For this review, take the finished solid that the model builds, in its own axes (mm). A direction names the side the tool comes from. Round coordinates to 2 decimals unless told otherwise and drop trailing zeros. Loops run counter-clockwise (first coordinate to the right, second up) from the corner with the lowest first, then second, coordinate; pieces in that order, holes last.
1) Insertion check: pin 1 (0.9 mm diameter, centred on y = 19.5, z = 12.5, fed in from -X); pin 2 (10 mm diameter, centred on y = 12.5, z = 10, fed in from +X) (3 decimals); pin 3 (5 mm diameter, centred on x = 31, y = 14.5, fed in from +Z). Each pin has a flat end and moves straight along its axis. Give the tip position at first contact, or say it passes through.
2) Take a section at A-A (z = 26.5). State the section outline as (x, y) points.
3) Mouldability with a two-part tool opening along Z and no side actions: class faces 1 (the cylindrical face through (71, 20.5, 12.6)), 2 (the flat face through (53, 13, 0)), 3 (the flat face through (53, 0, 12)) as pulls with the +Z half, pulls with the -Z half, needs draft (parallel to the pull), parting line crosses it, or undercut.
4) Tool access review of faces 4 (the cylindrical face through (71, 4.5, 12.4)), 5 (the cylindrical face through (33, 20.5, 12.6)), 6 (the cylindrical face through (66.61, 9.44, 23.16)), 7 (the flat face through (74, 21, 35)): name each direction out of +Z, -Z, +X, -X, +Y, -Y from which nothing blocks a thin tool from reaching the whole face with its end or side.
5) Wall thickness on L1, parallel to X at y = 13, z = 23; L2, parallel to Y at x = 11, z = 12.5; L3, parallel to Y at x = -5, z = 12.5: over which ranges is each line inside the solid? List them lowest first.
6) Take a section at D-D (y = 12.5). Give the number of separate pieces and of enclosed holes in the cut face, then the cut area to 3 significant figures.
7) Take a section at B-B (x = 17). State the section outline as (y, z) points, then the cut area to 3 significant figures.
8) Take a section at C-C (x = 79.5). State the section outline as (y, z) points.
```python
from build123d import *

# Parameters (mm, degrees)
SZKIC1_W                    = 52
SZKIC1_H                    = 25
DODANIE_WYCI_GNI_CIE1_DEPTH = 25
SZKIC1_3_R                  = 10
DODANIE_WYCI_GNI_CIE2_DEPTH = 35
SZKIC2_R                    = 10
DODANIE_WYCI_GNI_CIE3_DEPTH = 15
SZKIC3_R                    = 8
WYTNIJ_WYCI_GNI_CIE1_DEPTH  = 50
SZKIC4_R                    = 8
WYTNIJ_WYCI_GNI_CIE2_DEPTH  = 31


with BuildPart() as part:
    # Szkic1 → Dodanie-wyci_gni_cie1 (new body)
    with BuildSketch(Plane.XY):
        with Locations((26, 12.5)):
            Rectangle(SZKIC1_W, SZKIC1_H)
    extrude(amount=DODANIE_WYCI_GNI_CIE1_DEPTH)

    # Szkic1_3 → Dodanie-wyci_gni_cie2 (add)
    with BuildSketch(Plane.XY):
        with Locations((30, 12.5)):
            Circle(SZKIC1_3_R)
    extrude(amount=DODANIE_WYCI_GNI_CIE2_DEPTH)

    # Szkic2 → Dodanie-wyci_gni_cie3 (add)
    with BuildSketch(Plane(origin=(0, 0, 0), x_dir=(0, 0, -1), z_dir=(1, 0, 0))):
        with Locations((-12.5, 12.5)):
            Circle(SZKIC2_R)
    extrude(amount=-DODANIE_WYCI_GNI_CIE3_DEPTH)

    # Szkic3 → Wytnij-wyci_gni_cie1 (cut)
    with BuildSketch(Plane.ZY.offset(15)):
        with Locations((12.5, 12.5)):
            Circle(SZKIC3_R)
    extrude(amount=-WYTNIJ_WYCI_GNI_CIE1_DEPTH, mode=Mode.SUBTRACT)

    # Szkic4 → Wytnij-wyci_gni_cie2 (cut)
    with BuildSketch(Plane.XY.offset(35)):
        with Locations((30, 12.5)):
            Circle(SZKIC4_R)
    extrude(amount=-WYTNIJ_WYCI_GNI_CIE2_DEPTH, mode=Mode.SUBTRACT)

    # Lustro1: part across plane


with BuildPart() as part_1:
    add(part.part)
    add(part.part.mirror(Plane(origin=(52, 0, 25), x_dir=(0, 0, 1), z_dir=(1, 0, 0))))


solid = part_1.part
```
Response:
1. pin 1: stops at x = 35
1. pin 2: stops at x = 67.755
1. pin 3: stops at z = 4
2. outline: circle Ø20 at (30, 12.5); circle Ø20 at (74, 12.5); hole circle Ø16 at (30, 12.5); hole circle Ø16 at (74, 12.5)
3. face 1: undercut
3. face 2: pulls with the -Z half
3. face 3: needs draft
4. face 4: +X
4. face 5: -X
4. face 6: +Z
4. face 7: +Z, +X, -X, +Y, -Y
5. L1: x = 0 to 22.02, 37.98 to 66.02, 81.98 to 104
5. L2: y = 0 to 4.5, 20.5 to 25
5. L3: y = 2.5 to 4.5, 20.5 to 22.5
6. separate pieces: 3
6. enclosed holes: 0
6. area: 1,420 mm2
7. outline: (0, 0) - (25, 0) - (25, 25) - (0, 25) - close; hole circle Ø16 at (12.5, 12.5)
7. area: 424 mm2
8. outline: (0, 0) - (25, 0) - (25, 25) - (20.85, 25) - (20.85, 35) - (18.31, 35) - (18.31, 18) arc R8 cw to (18.31, 7) - (18.31, 4) - (6.69, 4) - (6.69, 7) arc R8 cw to (6.69, 18) - (6.69, 35) - (4.15, 35) - (4.15, 25) - (0, 25) - close
